Design review of the part built by this model. Coordinates are the model's own, in mm. A direction names the side the tool comes from. Round coordinates to 2 decimals unless told otherwise and drop trailing zeros. Write each loop counter-clockwise with the first axis right and the second up, starting at its lowest first coordinate (ties: lowest second). Pieces come first, ordered by that corner, then holes. Notation, with made-up numbers: M 39.5,-9.75 L 63.5,-9.75 A13 ccw 63.5,8.25 Z; hole C 69,71.25 d4. An arc over 180 degrees is marked long. One line per question, with ' | ' between items. Start each with the question number.
Item 1: Add section A-A, the plane y = 28. State the section outline as (x, z) points (3 decimals).
Item 2: Draft analysis for pull direction Y (two halves, no side actions). For faces 1 (the face through (0, 0, 0)), 2 (the face through (5.202, 10.135, -17.842)), 3 (the face through (-1.82, 36.54, 13.85)), 4 (the face through (-13.06, 26.82, -12.96)), state which applies: released by +Y, released by -Y, zero draft, split by the parting line, or undercut.
Item 3: Insertion check: pin 1 Ø10 at (x, y) = (12, 23) entering from +Z; pin 2 Ø8.5 at (y, z) = (9.906, 0) entering from -X; pin 3 Ø3 at (y, z) = (11, 16) entering from +X. Each pin has a flat end and moves straight along its axis. Give the tip position at first contact, or say it passes through.
Item 4: Add section D-D, the plane y = 58. State the section outline as (x, z) points.
Item 5: Machinability: for faces 5 (the face through (-17.756, 26.824, 4.829)), 6 (the face through (-4.16, 16.44, -17.16)), 7 (the face through (4.829, 26.824, 17.756)), 8 (the face through (15.748, 40.368, 4.959)), which of the approach directions +Z, -Z, +X, -X, +Y, -Y give a long, thin tool a straight path to every point of the face, cutting with its end or side? Answer none if there is none.
Item 6: For L1, parallel to Y at x = 0, z = -17.75; L2, parallel to Y at x = 0, z = 16; L3, parallel to Y at x = -4.5, z = 17, list the stretches that pass through material, from the lowest coordinate up.
Item 7: Add section B-B, the plane z = 18. State the section outline as (x, y) points.
```python
from build123d import *

# Parameters (mm, degrees)
CUT_EXTRUDE1_START  = -14.224
CUT_EXTRUDE1_DEPTH  = 14.224
BOSS_EXTRUDE1_START = -2.344817
SKETCH3_R           = 7.747
SKETCH3_R_2         = 5.207
BOSS_EXTRUDE1_DEPTH = 11.234817
CIRPATTERN1_COUNT   = 4
SKETCH4_R           = 7.747
CUT_EXTRUDE2_DEPTH  = 3.81
FILLET1_R           = 2.54


with BuildPart() as part:
    # Sketch1 → Revolve1 (revolve)
    with BuildSketch(Plane.XY):
        Polygon((0, 73.914), (13.97, 73.914), (13.97, 41.656), (16.51, 41.656), (16.51, 39.116), (13.97, 39.116), (13.97, 34.036), (19.05, 34.036), (19.05, 19.812), (13.97, 19.812), (13.97, 0), (0, 0), align=None)
    revolve(axis=Axis((0, 73.914, 0), (0, -1, 0)))

    # Sketch2 → Cut-Extrude1 (cut)
    with BuildSketch(Plane(origin=(0, 34.036, 0), x_dir=(1, 0, 0), z_dir=(0, 1, 0)).offset(CUT_EXTRUDE1_START)):
        with BuildLine():
            ThreePointArc((9.525, 16.497783942), (4.930502809, 18.400886991), (0, 19.05))
            Line((0, 19.05), (9.525, 16.497783942))
        make_face()
        with BuildLine():
            Line((-9.525, 16.497783942), (0, 19.05))
            ThreePointArc((0, 19.05), (-4.930502809, 18.400886991), (-9.525, 16.497783942))
        make_face()
        with BuildLine():
            Line((-16.497783942, 9.525), (-9.525, 16.497783942))
            ThreePointArc((-9.525, 16.497783942), (-13.470384182, 13.470384182), (-16.497783942, 9.525))
        make_face()
        with BuildLine():
            ThreePointArc((16.497783942, 9.525), (13.470384182, 13.470384182), (9.525, 16.497783942))
            Line((9.525, 16.497783942), (16.497783942, 9.525))
        make_face()
        with BuildLine():
            Line((-19.05, 0), (-16.497783942, 9.525))
            ThreePointArc((-16.497783942, 9.525), (-18.400886991, 4.930502809), (-19.05, 0))
        make_face()
        with BuildLine():
            ThreePointArc((19.05, 0), (18.400886991, 4.930502809), (16.497783942, 9.525))
            Line((16.497783942, 9.525), (19.05, 0))
        make_face()
        with BuildLine():
            Line((-16.497783942, -9.525), (-19.05, 0))
            ThreePointArc((-19.05, 0), (-18.400886991, -4.930502809), (-16.497783942, -9.525))
        make_face()
        with BuildLine():
            ThreePointArc((16.497783942, -9.525), (18.400886991, -4.930502809), (19.05, 0))
            Line((19.05, 0), (16.497783942, -9.525))
        make_face()
        with BuildLine():
            Line((-9.525, -16.497783942), (-16.497783942, -9.525))
            ThreePointArc((-16.497783942, -9.525), (-13.470384182, -13.470384182), (-9.525, -16.497783942))
        make_face()
        with BuildLine():
            ThreePointArc((9.525, -16.497783942), (13.470384182, -13.470384182), (16.497783942, -9.525))
            Line((16.497783942, -9.525), (9.525, -16.497783942))
        make_face()
        with BuildLine():
            Line((0, -19.05), (-9.525, -16.497783942))
            ThreePointArc((-9.525, -16.497783942), (-4.930502809, -18.400886991), (0, -19.05))
        make_face()
        with BuildLine():
            ThreePointArc((0, -19.05), (4.930502809, -18.400886991), (9.525, -16.497783942))
            Line((9.525, -16.497783942), (0, -19.05))
        make_face()
    extrude(amount=CUT_EXTRUDE1_DEPTH, mode=Mode.SUBTRACT)

    # Sketch3 → Boss-Extrude1 (add)
    with BuildSketch(Plane.XY.offset(13.97).offset(BOSS_EXTRUDE1_START)):
        with Locations((0, 9.906)):
            Circle(SKETCH3_R)
        with Locations((0, 9.906)):
            Circle(SKETCH3_R_2, mode=Mode.SUBTRACT)
    boss_extrude1 = extrude(amount=BOSS_EXTRUDE1_DEPTH)

    # CirPattern1: Boss-Extrude1 ×4 about axis
    cirpattern1_axis = Axis((0, 0, 0), (0, 1, 0))
    for i in range(1, CIRPATTERN1_COUNT):
        add(boss_extrude1.rotate(cirpattern1_axis, i * 360 / CIRPATTERN1_COUNT))

    # Sketch4 → Cut-Extrude2 (cut)
    with BuildSketch(Plane(origin=(22.86, 0, 0), x_dir=(0, 0, -1), z_dir=(1, 0, 0))):
        with Locations((0, 9.906)):
            Circle(SKETCH4_R)
    cut_extrude2 = extrude(amount=-CUT_EXTRUDE2_DEPTH, mode=Mode.SUBTRACT)

    # Mirror2: Cut-Extrude2 across plane
    add(cut_extrude2.mirror(Plane(origin=(0, 0, 0), x_dir=(0, 0, 1), z_dir=(1, 0, 0))), mode=Mode.SUBTRACT)

    # Fillet1
    fillet1_edges = [part.edges().sort_by_distance(p)[0] for p in [
        (-13.97, 73.914, 0),
    ]]
    fillet(fillet1_edges, radius=FILLET1_R)


solid = part.part
```
Computed values:
1) outline: M -19.05,0 L -16.498,-9.525 L -9.525,-16.498 L 0,-19.05 L 9.525,-16.498 L 16.498,-9.525 L 19.05,0 L 16.498,9.525 L 9.525,16.498 L 0,19.05 L -9.525,16.498 L -16.498,9.525 Z
2) face 1: released by -Y | face 2: undercut | face 3: undercut | face 4: zero draft
3) pin 1: stops at z = 17.17 | pin 2: stops at x = -13.97 | pin 3: stops at x = 7.75
4) outline: C 0,0 d27.94
5) face 5: +Z, -X, +Y | face 6: -Z | face 7: +Z, +X, +Y | face 8: +Y
6) L1: y = 2.16 to 4.7, 15.11 to 17.65, 19.81 to 34.04 | L2: y = 2.16 to 4.7, 15.11 to 17.65, 19.81 to 34.04, 39.12 to 41.66 | L3: y = 3.6 to 7.29, 12.53 to 16.21, 19.81 to 34.04
7) outline: C 0,9.91 d15.49; M -3.92,19.81 L 3.92,19.81 L 3.92,34.04 L -3.92,34.04 Z; hole C 0,9.91 d10.41
